Geometry check sheet. Reference: the model listing, model coordinates, mm. Face numbers are marked on the shaded views. A direction names the side the tool comes from. Coordinates: 2 decimals unless noted, no trailing zeros. Write each loop counter-clockwise with the first axis right and the second up, starting at its lowest first coordinate (ties: lowest second). Pieces come first, ordered by that corner, then holes. Notation, with made-up numbers: (70.25, -33.75) -> (102.25, -33.75) arc R26 cw to (102.25, -6.75) -> close; hole circle Ø2 at (16, 77). An arc over 180 degrees is marked (long way). One line per question, with ' | ' between items.
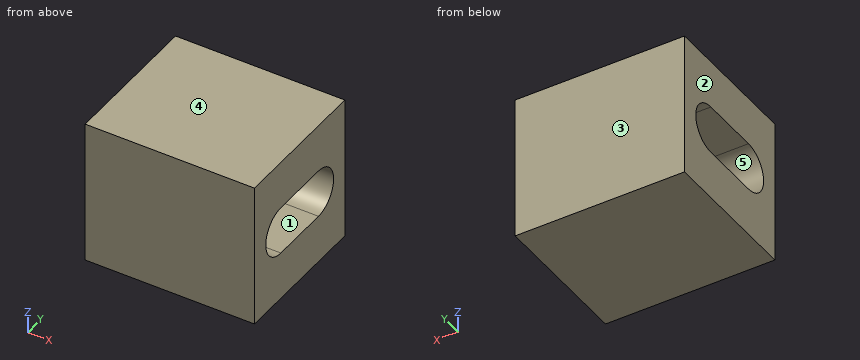
Autodesk Inventor part; units mm, degrees
ref_plane "YZ Plane" through (0, 0, 0) normal (1, 0, 0) x (0, 1, 0)
ref_plane "XZ Plane" through (0, 0, 0) normal (0, 1, 0) x (-1, 0, 0)
ref_plane "XY Plane" through (0, 0, 0) normal (0, 0, 1) x (1, 0, 0)
sketch "스케치1" plane through (0, 0, 0) normal (0, 1, 0) x (-1, 0, 0)
  line L0 (7, 6) -> (-7, 6)
  line L1 (-7, 6) -> (-7, -6)
  line L2 (-7, -6) -> (7, -6)
  line L3 (7, -6) -> (7, 6)
  line L4 (7, 6) -> (-7, -6) construction
  line L5 (-7, 6) -> (7, -6) construction
  point P0 (0, 0)
  dimension "d0" = 14
  dimension "d1" = 12
extrude "돌출1" add sketch "스케치1" along normal mid plane 12
sketch "스케치3" plane through (7, -6, -6) normal (1, 0, 0) x (0, 0, -1)
  line L0 (-14.9639, 6) -> (4.1102, 6) construction
  line L1 (-6, -0.8058) -> (-6, 13.755)
  line L2 (-12, 12) -> (0, 12)
  line L3 (-14.4911, 8.5) -> (7.0888, 8.5)
  arc A0 (-4, 8.5) -> (-8, 8.5) centre (-6, 8.5) ccw
  arc A1 (-8, 3.5) -> (-4, 3.5) centre (-6, 3.5) ccw
  line L4 (-8, 3.5) -> (-8, 8.5)
  line L5 (-4, 3.5) -> (-4, 8.5)
  point P0 (-6, 6)
  dimension "d8" = 6
  dimension "d9" = 5
  dimension "d10" = 4
extrude "돌출2" cut sketch "스케치3" against normal up to surface (14 mm away)
properties part number "multiblock_12x12x14" material "폴리스티렌"
1. Tool access check on the marked faces 1 and 2. Record the directions out of +Z, -Z, +X, -X, +Y, -Y that give a thin tool (end or side, any length) a straight path to the whole face; none if there is none.
Worked answers:
face 1: +X, -X | face 2: +Z, -Z, -X, +Y, -Y
2. Material ranges on line 1 (Z direction, x = -5.5, y = -1.25); line 2 (Z direction, x = -4, y = 3.75); line 3 (Y direction, x = 0.25, z = -1.5), recorded low to high. Write a range as from..to.
Worked answers:
line 1: -6..-2, 2..6 | line 2: -6..-1.56, 1.56..6 | line 3: -6..-3.82, 3.82..6
3. Cross-section at B-B on y = 1.5. Record the boundary of the cut face in (x, z), and give its area (3 significant figures).
Worked answers:
outline: (-7, -6) -> (7, -6) -> (7, -2) -> (-7, -2) -> close; (-7, 2) -> (7, 2) -> (7, 6) -> (-7, 6) -> close | area: 112 mm²
4. Cross-section at A-A on z = 0. Record the boundary of the cut face in (x, y), and give its area (3 significant figures).
Worked answers:
outline: (-7, -6) -> (7, -6) -> (7, -4.5) -> (-7, -4.5) -> close; (-7, 4.5) -> (7, 4.5) -> (7, 6) -> (-7, 6) -> close | area: 42.0 mm²
5. Cross-section at C-C on x = 4. Record the boundary of the cut face in (y, z), and give its area (3 significant figures).
Worked answers:
outline: (-6, -6) -> (6, -6) -> (6, 6) -> (-6, 6) -> close; hole (-2.5, -2) -> (2.5, -2) arc R2 ccw to (2.5, 2) -> (-2.5, 2) arc R2 ccw to start | area: 111 mm²
6. Mould release check, pull along Z, two halves, no side actions. Record for the marked faces 3, 4 and 5: released by +Z, released by -Z, zero draft, split by the parting line, or undercut.
Worked answers:
face 3: zero draft | face 4: released by +Z | face 5: undercut
